Part model, mm, in its own coordinate system. A direction names the side the tool comes from. Coordinates: 2 decimals unless noted, no trailing zeros. Loops run counter-clockwise (first coordinate to the right, second up) from the corner with the lowest first, then second, coordinate; pieces in that order, holes last.
```python
from build123d import *

# Parameters (mm, degrees)
BOX006_W                   = 3
BOX006_H                   = 5.7
BOX006_DEPTH               = 0.35
BOX007_W                   = 2
BOX007_H                   = 5.7
BOX007_DEPTH               = 0.35
BOX005_W                   = 2
BOX005_H                   = 5.7
BOX005_DEPTH               = 0.35
EXTRUDE001_DEPTH           = 5.7
EXTRUDE002_DEPTH           = 5.7
EXTRUDE002_PLACEMENT_ANGLE = 90
EXTRUDE003_DEPTH           = 5.7
EXTRUDE003_PLACEMENT_ANGLE = 90
EXTRUDE_DEPTH              = 5.7
CYLINDER001_R              = 1
CYLINDER001_DEPTH          = 10
CYLINDER_R                 = 1
CYLINDER_DEPTH             = 10
BOX_W                      = 3.4
BOX_H                      = 5.7
BOX_DEPTH                  = 1.9
BOX001_W                   = 12.6
BOX001_H                   = 5.7
BOX001_DEPTH               = 2.7


with BuildPart() as cube006:
    # Box006 → Box006 (new body)
    with BuildSketch(Plane(origin=(4.8, 0, 0), x_dir=(1, 0, 0), z_dir=(0, 0, 1))):
        with Locations((1.5, 2.85)):
            Rectangle(BOX006_W, BOX006_H)
    extrude(amount=BOX006_DEPTH)


with BuildPart() as cube007:
    # Box007 → Box007 (new body)
    with BuildSketch(Plane(origin=(10.6, 0, 0), x_dir=(1, 0, 0), z_dir=(0, 0, 1))):
        with Locations((1, 2.85)):
            Rectangle(BOX007_W, BOX007_H)
    extrude(amount=BOX007_DEPTH)


with BuildPart() as cube005:
    # Box005 → Box005 (new body)
    with BuildSketch(Plane.XY):
        with Locations((1, 2.85)):
            Rectangle(BOX005_W, BOX005_H)
    extrude(amount=BOX005_DEPTH)


with BuildPart() as extrude001:
    # Sketch001 → Extrude001 (new body)
    with BuildSketch(Plane.XZ):
        Polygon((0, 0), (0, 0.35), (0.35, 0), align=None)
    extrude(amount=-EXTRUDE001_DEPTH)


with BuildPart() as extrude001_1:
    # Extrude001 placement: moved
    add(extrude001.part.moved(Location((7.8, 0, 0))))


with BuildPart() as extrude002:
    # Sketch002 → Extrude002 (new body)
    with BuildSketch(Plane.XZ):
        Polygon((0, 0), (0, 0.35), (0.35, 0), align=None)
    extrude(amount=-EXTRUDE002_DEPTH)


with BuildPart() as extrude002_1:
    # Extrude002 placement: moved
    add(extrude002.part.moved(Location((4.8, 0, 0))).rotate(Axis((4.8, 0, 0), (0, -1, 0)), EXTRUDE002_PLACEMENT_ANGLE))


with BuildPart() as extrude003:
    # Sketch003 → Extrude003 (new body)
    with BuildSketch(Plane.XZ):
        Polygon((0, 0), (0, 0.35), (0.35, 0), align=None)
    extrude(amount=-EXTRUDE003_DEPTH)


with BuildPart() as extrude003_1:
    # Extrude003 placement: moved
    add(extrude003.part.moved(Location((10.6, 0, 0))).rotate(Axis((10.6, 0, 0), (0, -1, 0)), EXTRUDE003_PLACEMENT_ANGLE))


with BuildPart() as extrude_body:
    # Sketch → Extrude (new body)
    with BuildSketch(Plane.XZ):
        Polygon((0, 0), (0, 0.35), (0.35, 0), align=None)
    extrude(amount=-EXTRUDE_DEPTH)


with BuildPart() as extrude_body_1:
    # Extrude placement: moved
    add(extrude_body.part.moved(Location((2, 0, 0))))


with BuildPart() as cylinder001:
    # Cylinder001 → Cylinder001 (new body)
    with BuildSketch(Plane(origin=(9.6, -2, 1.5), x_dir=(1, 0, 0), z_dir=(0, 1, 0))):
        Circle(CYLINDER001_R)
    extrude(amount=CYLINDER001_DEPTH)


with BuildPart() as cylinder:
    # Cylinder → Cylinder (new body)
    with BuildSketch(Plane(origin=(3, -2, 1.5), x_dir=(1, 0, 0), z_dir=(0, 1, 0))):
        Circle(CYLINDER_R)
    extrude(amount=CYLINDER_DEPTH)


with BuildPart() as cube:
    # Box → Box (new body)
    with BuildSketch(Plane(origin=(4.6, 0, 0.8), x_dir=(1, 0, 0), z_dir=(0, 0, 1))):
        with Locations((1.7, 2.85)):
            Rectangle(BOX_W, BOX_H)
    extrude(amount=BOX_DEPTH)


with BuildPart() as cut011:
    # Box001 → Box001 (new body)
    with BuildSketch(Plane.XY):
        with Locations((6.3, 2.85)):
            Rectangle(BOX001_W, BOX001_H)
    extrude(amount=BOX001_DEPTH)

    # Cut002: cut Cube
    add(cube.part, mode=Mode.SUBTRACT)

    # Cut003: cut Cylinder
    add(cylinder.part, mode=Mode.SUBTRACT)

    # Cut004: cut Cylinder001
    add(cylinder001.part, mode=Mode.SUBTRACT)

    # Cut005: cut Extrude body
    add(extrude_body_1.part, mode=Mode.SUBTRACT)

    # Cut006: cut Extrude003
    add(extrude003_1.part, mode=Mode.SUBTRACT)

    # Cut007: cut Extrude002
    add(extrude002_1.part, mode=Mode.SUBTRACT)

    # Cut008: cut Extrude001
    add(extrude001_1.part, mode=Mode.SUBTRACT)

    # Cut009: cut Cube005
    add(cube005.part, mode=Mode.SUBTRACT)

    # Cut010: cut Cube007
    add(cube007.part, mode=Mode.SUBTRACT)

    # Cut011: cut Cube006
    add(cube006.part, mode=Mode.SUBTRACT)


solid = cut011.part
```
Q1. Mould opens along X. For faces 1 (the flat face through (6, 3, 0.35)), 2 (the flat face through (2, 3, 2.7)), 3 (the flat face through (12.6, 3, 2)), 4 (the flat face through (0, 3, 2)) say: released by +X, released by -X, zero draft, split by the parting line, or undercut.
Q2. Saw through at C-C (y = 2.7). List the corners of the cut face in (x, z).
Q3. Saw through at B-B (z = 1.5). List the corners of the cut face in (x, y), plus the area to 3 significant figures.
Q4. Drop flat-ended pins along their axis: P1, Ø1.5, axis at x = 6, y = 2, coming from the -Z side; P2, Ø1, axis at x = 6, y = 4.5, coming from the +Z side. Give the stop position or say it passes through.
Q5. Tool access for faces 5 (the flat face through (9, 3, 0)), 6 (the flat face through (4.6, 3, 2)), 7 (the flat face through (1, 3, 0.35)), 8 (the flat face through (12, 3, 0.35)): list every direction of +Z, -Z, +X, -X, +Y, -Y with a clear straight run to the whole face (end or side of a thin tool).
Q6. Saw through at D-D (x = 3). List the corners of the cut face in (y, z).
Q7. Saw through at A-A (x = 9). List the corners of the cut face in (y, z).
Q8. Probe line 1 (Z direction, x = 3, y = 2.1); line 2 (X direction, y = 1.3, z = 1.85); line 3 (X direction, y = 1.25, z = 2.35). List the from-to ranges inside material, lowest first.
Checked values:
1. face 1: undercut
1. face 2: zero draft
1. face 3: released by +X
1. face 4: released by -X
2. outline: (0, 0.35) - (2, 0.35) - (2.35, 0) - (4.45, 0) - (4.8, 0.35) - (7.8, 0.35) - (8.15, 0) - (10.25, 0) - (10.6, 0.35) - (12.6, 0.35) - (12.6, 2.7) - (8, 2.7) - (8, 0.8) - (4.6, 0.8) - (4.6, 2.7) - (0, 2.7) - close; hole circle Ø2 at (3, 1.5); hole circle Ø2 at (9.6, 1.5)
3. outline: (0, 0) - (2, 0) - (2, 5.7) - (0, 5.7) - close; (4, 0) - (4.6, 0) - (4.6, 5.7) - (4, 5.7) - close; (8, 0) - (8.6, 0) - (8.6, 5.7) - (8, 5.7) - close; (10.6, 0) - (12.6, 0) - (12.6, 5.7) - (10.6, 5.7) - close
3. area: 29.6 mm2
4. P1: stops at z = 0.35
4. P2: stops at z = 0.8
5. face 5: -Z, +X, -X, +Y, -Y
5. face 6: +Z, +Y, -Y
5. face 7: -Z, -X, +Y, -Y
5. face 8: -Z, +X, +Y, -Y
6. outline: (0, 0) - (5.7, 0) - (5.7, 0.5) - (0, 0.5) - close; (0, 2.5) - (5.7, 2.5) - (5.7, 2.7) - (0, 2.7) - close
7. outline: (0, 0) - (5.7, 0) - (5.7, 0.7) - (0, 0.7) - close; (0, 2.3) - (5.7, 2.3) - (5.7, 2.7) - (0, 2.7) - close
8. line 1: z = 0 to 0.5, 2.5 to 2.7
8. line 2: x = 0 to 2.06, 3.94 to 4.6, 8 to 8.66, 10.54 to 12.6
8. line 3: x = 0 to 2.47, 3.53 to 4.6, 8 to 9.07, 10.13 to 12.6
